Input: part model. Units: mm. Frame: model coordinates. Coordinates: 2 decimals unless noted, no trailing zeros. Loops run counter-clockwise (first coordinate to the right, second up) from the corner with the lowest first, then second, coordinate; pieces in that order, holes last. Notation, with made-up numbers: (57.5, 12) - (115.5, 12) arc R18 ccw to (115.5, 28) - close; hole circle Ø11 at (89, 61.25). An arc over 180 degrees is marked (long way). Use a Markdown table: item, result. Add a question column.
1. Section query B-B on x = 0.25. Return the cut outline in (y, z), then the cut area to 3 significant figures.
2. Contact query for flat-ended pins moving along their axis: P1, Ø12, axis at y = 0, z = 0, coming from the +X side; P2, Ø3, axis at x = -3.5, z = 2, coming from the +Y side; P3, Ø1.5, axis at x = 1, z = 7, coming from the -Y side. Output: stop coordinate, or through.
3. Section query A-A on x = -4.75. Return the cut outline in (y, z).
4. Draft query along Z for faces 1 (the face through (4.392, 11.547, 4.788)), 2 (the face through (-6, -6, 9)), 3 (the face through (0.08, -2.17, 9.76)). Return one class per face: released by +Z, released by -Z, zero draft, split by the parting line, or undercut.
5. Ray query, L1, parallel to Z at x = 1.25, y = -2; L2, parallel to Z at x = -2.5, y = 0; L3, parallel to Y at x = -4.25, z = -7.75. Return the intervals inside material, ascending. Write a range as [from, to].
```python
from build123d import *

# Parameters (mm, degrees)
FILLET1_R = 0.6
FILLET2_R = 0.5


with BuildPart() as part:
    # Sketch1 → Revolve1 (revolve)
    with BuildSketch(Plane.XY):
        with BuildLine():
            Line((-6, 12.5), (-6, 10))
            Line((-6, 10), (6, 10))
            Line((6, 10), (6, 12.5))
            Line((6, 12.5), (2.645751311, 12.5))
            ThreePointArc((2.645751311, 12.5), (0, 11.5), (-2.645751311, 12.5))
            Line((-2.645751311, 12.5), (-6, 12.5))
        make_face()
    revolve(axis=Axis((44.126443973, 0, 0), (-1, 0, 0)))

    # Fillet1
    fillet1_edges = [part.edges().sort_by_distance(p)[0] for p in [
        (6, -10, 0),
        (-6, -10, 0),
    ]]
    fillet(fillet1_edges, radius=FILLET1_R)

    # Fillet2
    fillet2_edges = [part.edges().sort_by_distance(p)[0] for p in [
        (2.645751311, -12.5, 0),
        (-2.645751311, -12.5, 0),
    ]]
    fillet(fillet2_edges, radius=FILLET2_R)


solid = part.part
```
Resolved:
| question | item | result |
|---|---|---|
| 1 | outline | circle Ø23.02 at (0, 0); hole circle Ø20 at (0, 0) |
| 1 | area | 102 mm² |
| 2 | P1 | through |
| 2 | P2 | y = 12.49 |
| 2 | P3 | y = -9.88 |
| 3 | outline | circle Ø25 at (0, 0); hole circle Ø20 at (0, 0) |
| 4 | face 1 | split by the parting line |
| 4 | face 2 | zero draft |
| 4 | face 3 | undercut |
| 5 | L1 | [-11.53, -9.8], [9.8, 11.53] |
| 5 | L2 | [-12.38, -10], [10, 12.38] |
| 5 | L3 | [-9.81, -6.32], [6.32, 9.81] |
